Source: CAD feature listing. Evaluate the final solid. Frame: model axes, mm. A direction names the side the tool comes from. Give positions to 0.01 mm unless a question says otherwise; leave off trailing zeros. Loops run counter-clockwise (first coordinate to the right, second up) from the corner with the lowest first, then second, coordinate; pieces in that order, holes last. Notation, with made-up numbers: M 12,39.5 L 16,39.5 A22 ccw 16,49.5 Z; hole C 80.25,13 d10. An arc over 180 degrees is marked long. Answer in a Markdown table with one row per item.
```python
from build123d import *

# Parameters (mm, degrees)
SKETCH_2_R          = 3
SKETCH_2_R_2        = 2
CUT_EXTRUDE_1_DEPTH = 1
SKETCH_3_R          = 2
EXTRUDE_1_DEPTH     = 0.5
SKETCH_5_R          = 1
EXTRUDE_3_DEPTH     = 5


with BuildPart() as part:
    # 草图1 → 旋转2 (revolve)
    with BuildSketch(Plane.XY):
        with BuildLine():
            Line((7.513582187, 0), (7.513582187, -4))
            ThreePointArc((7.513582187, -4), (16.013582187, -4.614003224), (24.513582187, -4))
            Line((24.513582187, -4), (24.513582187, 0))
            Line((24.513582187, 0), (7.513582187, 0))
        make_face()
    revolve(axis=Axis((7.513582187, 0, 0), (1, 0, 0)))

    # 草图2 → 切除-拉伸1 (cut)
    with BuildSketch(Plane.ZY.offset(-7.513582187)):
        Circle(SKETCH_2_R)
        Circle(SKETCH_2_R_2, mode=Mode.SUBTRACT)
    cut_extrude_1 = extrude(amount=-CUT_EXTRUDE_1_DEPTH, mode=Mode.SUBTRACT)

    # 草图3 → 凸台-拉伸1 (add)
    with BuildSketch(Plane.ZY.offset(-7.513582187)):
        Circle(SKETCH_3_R)
    extrude_1 = extrude(amount=EXTRUDE_1_DEPTH)

    # 草图5 → 凸台-拉伸3 (add)
    with BuildSketch(Plane.ZY.offset(-7.013582187)):
        Circle(SKETCH_5_R)
    extrude_3 = extrude(amount=EXTRUDE_3_DEPTH)

    # 镜向4: 切除-拉伸1, 凸台-拉伸1, 凸台-拉伸3 across plane
    add(cut_extrude_1.mirror(Plane.ZY.offset(-16.013582187)), mode=Mode.SUBTRACT)
    add(extrude_1.mirror(Plane.ZY.offset(-16.013582187)))
    add(extrude_3.mirror(Plane.ZY.offset(-16.013582187)))


solid = part.part
```
Q1. Ray query, probe 1 along Y at (x, z) = (7.9, 0); probe 2 along Y at (x, z) = (24.2, 0); probe 3 along X at (y, z) = (3.5, 1.5). Return the intervals inside material, ascending. Write a range as from..to.
Values follow:
| item | result |
|---|---|
| probe 1 | -4.05..-3, -2..2, 3..4.05 |
| probe 2 | -4.04..-3, -2..2, 3..4.04 |
| probe 3 | 7.51..24.51 |
Q2. Contact query for flat-ended pins moving along their axis: pin 1 Ø2 at (x, z) = (10.5, 0.5) entering from +Y; pin 2 Ø5 at (x, z) = (8, 2.5) entering from +Y; pin 3 Ø5 at (x, z) = (20, 1) entering from -Y. Output: stop coordinate, or through.
Values follow:
| item | result |
|---|---|
| pin 1 | y = 4.43 |
| pin 2 | y = 4.23 |
| pin 3 | y = -4.59 |
Q3. Reachability of faces 1 (the flat face through (23.514, -2, 1)), 2 (the flat face through (2.014, 0, 0)), 3 (the cylindrical face through (8, -2, 0)) from +Z, -Z, +X, -X, +Y, -Y: full face, straight path, thin tool, end or side. Return the list, or none.
Values follow:
| item | result |
|---|---|
| face 1 | +X |
| face 2 | +Z, -Z, -X, +Y, -Y |
| face 3 | -X |
Q4. Section query A-A (x = 4.25). Output: boundary loops of the cut face in (y, z).
Values follow:
| item | result |
|---|---|
| outline | C 0,0 d2 |
Q5. Mould query, pull axis Y, two halves, no side actions, for faces 4 (the flat face through (25.014, -1, 1)), 5 (the cylindrical face through (27, -1, 0)), 6 (the flat face through (8.514, -2, 1)). Classes: +Y half, -Y half, draft (parallel to the pull), parting line (faces both ways), or undercut.
Values follow:
| item | result |
|---|---|
| face 4 | draft |
| face 5 | parting line |
| face 6 | undercut |
